Input: part model. Units: mm. Frame: model coordinates. A direction names the side the tool comes from. Give positions to 0.01 mm unless a question says otherwise; leave off trailing zeros. Loops run counter-clockwise (first coordinate to the right, second up) from the corner with the lowest first, then second, coordinate; pieces in that order, holes last. Notation, with made-up numbers: (-9.5, 87) - (14.5, 87) arc R28 ccw to (14.5, 125) - close; hole circle Ø10 at (-1, -7.75). An arc over 180 degrees is marked (long way). Answer as a JSON object with one key per item and string values. Group by question number.
(1) Mould query, pull axis X, two halves, no side actions, for faces 1 (the cylindrical face through (58.203, 6.014, -2.028)), 2 (the cylindrical face through (-153.78, 278.05, 2.84)), 3 (the flat face through (-143, 0, 0)), 4 (the flat face through (161, 278, 50)). Classes: +X half, -X half, draft (parallel to the pull), parting line (faces both ways), or undercut.
(2) Section query D-D (z = 9.5). Return loops of the section in (x, y), plus the area to 3 significant figures.
(3) Section query C-C (x = 99). Return loops of the section in (y, z), plus the area to 3 significant figures.
(4) Pin query (flat end, axial travel): P1, Ø2, axis at y = 85, z = -1.5, coming from the -X side; P2, Ø2, axis at x = -9, z = -2.5, coming from the -Y side; P3, Ø5, axis at x = -70, y = 387, coming from the +Z side. Return the tip coordinate at first contact, or that it passes through.
(5) Material intervals for L1, parallel to X at y = 344.5, z = 27.5; L2, parallel to X at y = 509, z = 18.5; L3, parallel to Z at x = 42, y = 537, sorted ascending.
(6) Section query A-A (z = 49.5). Return loops of the section in (x, y), plus the area to 3 significant figures.
(7) Section query B-B (y = 491). Return loops of the section in (x, z).
(8) Access query for faces 5 (the cylindrical face through (-58.203, 6.014, -2.028)), 6 (the cylindrical face through (154.16, 278.05, 3.22)), 7 (the flat face through (-2, 278, 0)). Directions: +Z, -Z, +X, -X, +Y, -Y. A direction counts if a zero-diameter tool reaches every point of the face in a straight line with its end or side. Return the directions, or none.
```python
from build123d import *

# Parameters (mm, degrees)
EXTRUDE_THIN1_DEPTH     = 564
CUT_EXTRUDE1_DEPTH      = 593.514134852
CUT_EXTRUDE1_DEPTH_BACK = 593.514134852
SKETCH2_W               = 105
SKETCH2_H               = 260.267111285
FILLET2_R               = 10
FILLET3_R               = 20


with BuildPart() as part:
    # Sketch1 → Extrude-Thin1 (new body)
    with BuildSketch(Plane(origin=(0, 0, 0), x_dir=(1, 0, 0), z_dir=(0, 1, 0))):
        with BuildLine():
            Line((-157, -80), (-157, -20))
            ThreePointArc((-157, -20), (-151.142135624, -5.857864376), (-137, 0))
            Line((-137, 0), (137, 0))
            ThreePointArc((137, 0), (151.142135624, -5.857864376), (157, -20))
            Line((157, -20), (157, -80))
            Line((157, -80), (161, -80))
            Line((161, -80), (161, -20))
            ThreePointArc((161, -20), (153.970562748, -3.029437252), (137, 4))
            Line((137, 4), (-137, 4))
            ThreePointArc((-137, 4), (-153.970562748, -3.029437252), (-161, -20))
            Line((-161, -20), (-161, -80))
            Line((-161, -80), (-157, -80))
        make_face()
    extrude(amount=EXTRUDE_THIN1_DEPTH)

    # Sketch2 → Cut-Extrude1 (cut, two sides: drawn at the far end of the back side and taken through both)
    with BuildSketch(Plane(origin=(0, 0, -4), x_dir=(-1, 0, 0), z_dir=(0, 0, -1)).offset(-CUT_EXTRUDE1_DEPTH_BACK)):
        with Locations((0, -10.133555642)):
            Rectangle(SKETCH2_W, SKETCH2_H)
    extrude(amount=CUT_EXTRUDE1_DEPTH + CUT_EXTRUDE1_DEPTH_BACK, mode=Mode.SUBTRACT)

    # Fillet2
    fillet2_edges = [part.edges().sort_by_distance(p)[0] for p in [
        (52.5, 120, -2),
        (-52.5, 120, -2),
    ]]
    fillet(fillet2_edges, radius=FILLET2_R)

    # Fillet3
    fillet3_edges = [part.edges().sort_by_distance(p)[0] for p in [
        (-52.5, 0, -2),
        (52.5, 0, -2),
    ]]
    fillet(fillet3_edges, radius=FILLET3_R)


solid = part.part
```
Recorded:
{
 "1": {"face 1": "undercut", "face 2": "-X half", "face 3": "draft", "face 4": "+X half"},
 "2": {"outline": "(-158.58, 0) - (-154.02, 0) - (-154.02, 564) - (-158.58, 564) - close; (154.02, 0) - (158.58, 0) - (158.58, 564) - (154.02, 564) - close", "area": "5,140 mm^2"},
 "3": {"outline": "(0, -4) - (564, -4) - (564, 0) - (0, 0) - close", "area": "2,260 mm^2"},
 "4": {"P1": "stops at x = -149.48", "P2": "stops at y = 120", "P3": "stops at z = 0"},
 "5": {"L1": "x = -161 to -157, 157 to 161", "L2": "x = -160.95 to -156.94, 156.94 to 160.95", "L3": "z = -4 to 0"},
 "6": {"outline": "(-161, 0) - (-157, 0) - (-157, 564) - (-161, 564) - close; (157, 0) - (161, 0) - (161, 564) - (157, 564) - close", "area": "4,510 mm^2"},
 "7": {"outline": "(-161, 20) arc R24 ccw to (-137, -4) - (137, -4) arc R24 ccw to (161, 20) - (161, 80) - (157, 80) - (157, 20) arc R20 cw to (137, 0) - (-137, 0) arc R20 cw to (-157, 20) - (-157, 80) - (-161, 80) - close"},
 "8": {"face 5": "+Z, -Z, -Y", "face 6": "-Z, +X, +Y, -Y", "face 7": "+Z, +Y, -Y"}
}
